Part model, mm, in its own coordinate system. Face numbers are marked on the shaded views. A direction names the side the tool comes from. Round coordinates to 2 decimals unless told otherwise and drop trailing zeros. Order: outer loops, then holes, each group sorted by start corner. A loop starts at its lowest first (then second) coordinate and runs counter-clockwise, first axis right, second up. Notation, with made-up numbers: (-31, 59.25) - (6, 59.25) arc R24 cw to (6, 72.25) - close; hole circle Ø3 at (72, -6.75). An arc over 180 degrees is marked (long way). Answer as a JSON object with one key per item and string values.
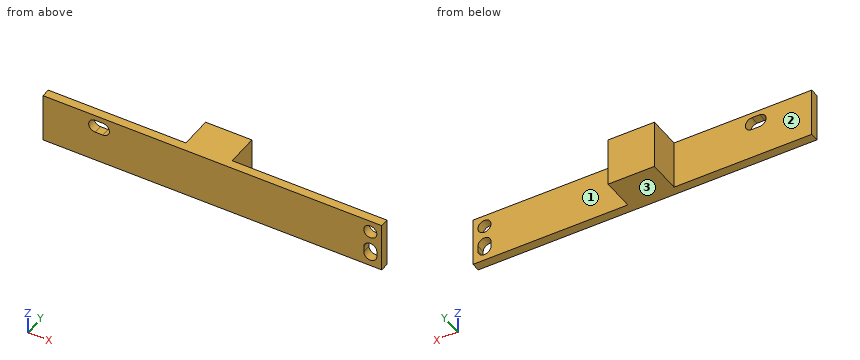
```python
from build123d import *

# Parameters (mm, degrees)
SKETCH1_W           = 62.2
SKETCH1_H           = 9
BOSS_EXTRUDE1_DEPTH = 1.6
SKETCH2_R           = 1.2
CUT_EXTRUDE1_DEPTH  = 2.6
SKETCH3_W           = 8.5
SKETCH3_H           = 9
BOSS_EXTRUDE2_DEPTH = 6


with BuildPart() as part:
    # Sketch1 → Boss-Extrude1 (new body)
    with BuildSketch(Plane(origin=(0, 0, 0), x_dir=(1, 0, 0), z_dir=(0, 1, 0))):
        with Locations((31.1, 4.5)):
            Rectangle(SKETCH1_W, SKETCH1_H)
    extrude(amount=BOSS_EXTRUDE1_DEPTH)

    # Sketch2 → Cut-Extrude1 (cut, through all)
    with BuildSketch(Plane(origin=(0, 1.6, 0), x_dir=(1, 0, 0), z_dir=(0, 1, 0))):
        with Locations((60.098236825, 2.147164508)):
            Circle(SKETCH2_R)
        with BuildLine():
            Line((9.591628176, 3.347164508), (10.991628176, 3.347164508))
            ThreePointArc((10.991628176, 3.347164508), (12.191628176, 2.147164508), (10.991628176, 0.947164508))
            Line((10.991628176, 0.947164508), (9.591628176, 0.947164508))
            ThreePointArc((9.591628176, 0.947164508), (8.391628176, 2.147164508), (9.591628176, 3.347164508))
        make_face()
        with BuildLine():
            Line((61.298236825, 6.7), (61.298236825, 5.7))
            ThreePointArc((61.298236825, 5.7), (60.098236825, 4.5), (58.898236825, 5.7))
            Line((58.898236825, 5.7), (58.898236825, 6.7))
            ThreePointArc((58.898236825, 6.7), (60.098236825, 7.9), (61.298236825, 6.7))
        make_face()
    extrude(amount=-CUT_EXTRUDE1_DEPTH, mode=Mode.SUBTRACT)

    # Sketch3 → Boss-Extrude2 (add)
    with BuildSketch(Plane(origin=(0, 1.6, 0), x_dir=(1, 0, 0), z_dir=(0, 1, 0))):
        with Locations((29.52, 4.5)):
            Rectangle(SKETCH3_W, SKETCH3_H)
    extrude(amount=BOSS_EXTRUDE2_DEPTH)


solid = part.part
```
Item 1: Drop flat-ended pins along their axis: P1, Ø4.5, axis at x = 47.5, z = -6, coming from the +Y side; P2, Ø1.5, axis at y = 5.5, z = -2, coming from the +X side. Give the stop position or say it passes through.
Taken from the geometry:
{"P1": "y = 1.6", "P2": "x = 33.77"}
Item 2: Cut at B-B (x = 50.5). Write the cut outline in (y, z), plus the area to 3 significant figures.
Taken from the geometry:
{"outline": "(0, -9) - (1.6, -9) - (1.6, 0) - (0, 0) - close", "area": "14.4 mm2"}
Item 3: Cut at A-A (y = 7). Write the cut outline in (x, z), plus the area to 3 significant figures.
Taken from the geometry:
{"outline": "(25.27, -9) - (33.77, -9) - (33.77, 0) - (25.27, 0) - close", "area": "76.5 mm2"}
Item 4: Probe L1, parallel to Y at x = 23.5, z = -1.5; L2, parallel to X at y = 6.75, z = -4.5; L3, parallel to X at y = 1.5, z = -7. List the from-to ranges inside material, lowest first. Write a range as from..to.
Taken from the geometry:
{"L1": "0..1.6", "L2": "25.27..33.77", "L3": "0..58.94, 61.26..62.2"}
Item 5: Tool access for the marked faces 1, 2 and 3: list every direction of +Z, -Z, +X, -X, +Y, -Y with a clear straight run to the whole face (end or side of a thin tool).
Taken from the geometry:
{"face 1": "+Z, -Z, +X, +Y", "face 2": "+Z, -Z, -X, +Y", "face 3": "-Z, +X, -X, +Y, -Y"}
